from build123d import *

# Parameters (mm, degrees)
SKETCH1_R           = 31.75
SKETCH1_R_2         = 15.875
BOSS_EXTRUDE1_DEPTH = 82.55
BOSS_EXTRUDE2_DEPTH = 82.55
SKETCH4_R           = 9.525
CUT_EXTRUDE1_DEPTH  = 82.55
SKETCH5_W           = 19.05
SKETCH5_H           = 82.55
BOSS_EXTRUDE3_DEPTH = 88.9
CHAMFER1_SIZE       = 25.4
CUT_EXTRUDE2_REACH  = 211.476
SKETCH6_R           = 15.875


with BuildPart() as part:
    # Sketch1 → Boss-Extrude1 (new body)
    with BuildSketch(Plane.XY):
        Circle(SKETCH1_R)
        Circle(SKETCH1_R_2, mode=Mode.SUBTRACT)
    extrude(amount=-BOSS_EXTRUDE1_DEPTH)

    # Sketch3 → Boss-Extrude2 (add)
    with BuildSketch(Plane.XY):
        Polygon((0.997093544, 31.734339515), (-81.552906456, 31.734339515), (-81.552906456, 12.684339515), (-29.106185443, 12.684339515), align=None)
        Polygon((0, -31.75), (95.25, -31.75), (95.25, -12.7), (29.099355663, -12.7), align=None)
    extrude(amount=-BOSS_EXTRUDE2_DEPTH)

    # Sketch4 → Cut-Extrude1 (cut)
    with BuildSketch(Plane(origin=(0, 31.734339515, 0), x_dir=(1, 0, 0), z_dir=(0, 1, 0))):
        with Locations(Location((-56.152906456, 63.5, 0), (0, 0, 180))):
            Circle(SKETCH4_R)
        with Locations(Location((-56.152906456, 19.05, 0), (0, 0, 180))):
            Circle(SKETCH4_R)
    extrude(amount=-CUT_EXTRUDE1_DEPTH, mode=Mode.SUBTRACT)

    # Sketch5 → Boss-Extrude3 (add)
    with BuildSketch(Plane(origin=(0, -12.7, 0), x_dir=(1, 0, 0), z_dir=(0, 1, 0))):
        with Locations((85.725, 41.275)):
            Rectangle(SKETCH5_W, SKETCH5_H)
    extrude(amount=BOSS_EXTRUDE3_DEPTH)

    # Chamfer1
    chamfer1_edges = [part.edges().sort_by_distance(p)[0] for p in [
        (85.725, 76.2, -82.55),
        (85.725, 76.2, 0),
    ]]
    chamfer(chamfer1_edges, length=CHAMFER1_SIZE)

    # Sketch6 → Cut-Extrude2 (cut, up to next)
    with BuildSketch(Plane(origin=(95.25, 0, 0), x_dir=(0, 0, -1), z_dir=(1, 0, 0)), mode=Mode.PRIVATE) as cut_extrude2_sk1:
        with Locations((41.275, 19.05)):
            Circle(SKETCH6_R)
    cut_extrude2_tool1 = extrude(cut_extrude2_sk1.sketch, amount=-CUT_EXTRUDE2_REACH, mode=Mode.PRIVATE) & part.part
    add(cut_extrude2_tool1.solids().sort_by_distance((95.25, 19.05, -41.275))[0], mode=Mode.SUBTRACT)


solid = part.part
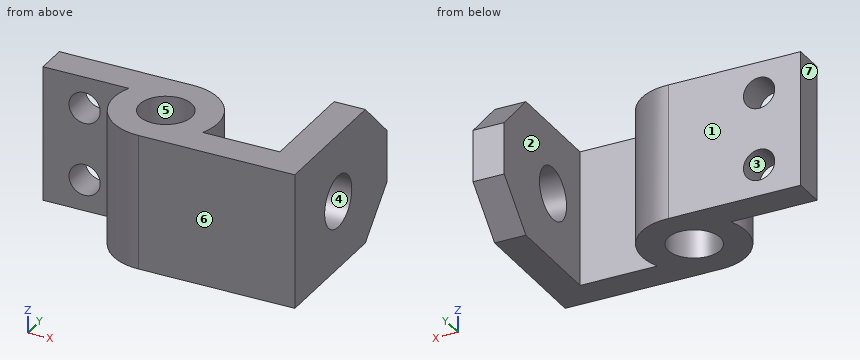
CAD build for the part. Positions are in the model's coordinates, mm. Face numbers are marked on the shaded views. A direction names the side the tool comes from. Round coordinates to 2 decimals unless told otherwise and drop trailing zeros. Write each loop counter-clockwise with the first axis right and the second up, starting at its lowest first coordinate (ties: lowest second). Pieces come first, ordered by that corner, then holes.
(1) 3-axis set-ups, long thin cutter, end or side, ignore diameter. For the marked faces 1, 2, 3 and 4: which of +Z, -Z, +X, -X, +Y, -Y reach the whole face in a straight line?
(2) Slice it at B-B, the plane z = -19.05. Write the cut outline in (x, y) (3 decimals).
(3) Slice it at A-A, the plane y = 19.05. Write the cut outline in (x, z) (3 decimals), and give its area (3 significant figures).
(4) Slice it at D-D, the plane z = -76.5. Write the cut outline in (x, y) (3 decimals).
(5) Slice it at C-C, the plane x = 11.5. Write the cut outline in (y, z), and give its area (3 significant figures).
(6) Probe line 1 along Y through (x, z) = (0, -54) (3 decimals); line 2 along X through (y, z) = (19.5, -16); line 3 along X through (y, z) = (3.5, -22). List the from-to ranges inside material, lowest first.
(7) Drop flat-ended pins along their axis: P1, Ø6, axis at x = -4.5, z = -52.5, coming from the +Y side; P2, Ø2, axis at x = -15.5, z = -39.5, coming from the -Y side; P3, Ø1, axis at x = -2, z = -39.5, coming from the -Y side. Give the stop position or say it passes through.
(8) Mould opens along X. For the marked faces 5, 6 and 7 say: pulls with the +X half, pulls with the -X half, needs draft (parallel to the pull), parting line crosses it, or undercut.
From the geometry:
1. face 1: +Z, -Z, -X, +Y
1. face 2: +Z, -Z, +Y
1. face 3: +Y, -Y
1. face 4: +X
2. outline: (-81.553, 12.684) - (-65.678, 12.684) - (-65.678, 31.734) - (-81.553, 31.734) - close; (-46.628, 12.684) - (-29.106, 12.684) arc R31.75 ccw to (0, -31.75) - (95.25, -31.75) - (95.25, 69.85) - (76.2, 69.85) - (76.2, -12.7) - (29.099, -12.7) arc R31.75 ccw to (-0.997, 31.734) - (-46.628, 31.734) - close; hole circle Ø31.75 at (0, 0)
3. outline: (-81.553, -82.55) - (25.4, -82.55) - (25.4, 0) - (-81.553, 0) - close; (76.2, -82.55) - (95.25, -82.55) - (95.25, -57.15) - (76.2, -57.15) - close; (76.2, -25.4) - (95.25, -25.4) - (95.25, 0) - (76.2, 0) - close; hole circle Ø19.05 at (-56.153, -63.5); hole circle Ø19.05 at (-56.153, -19.05)
3. area: 9,230 mm2
4. outline: (-81.553, 12.684) - (-29.106, 12.684) arc R31.75 ccw to (0, -31.75) - (95.25, -31.75) - (95.25, 56.85) - (76.2, 56.85) - (76.2, -12.7) - (29.099, -12.7) arc R31.75 ccw to (-0.997, 31.734) - (-81.553, 31.734) - close; hole circle Ø31.75 at (0, 0)
5. outline: (-31.75, -82.55) - (-10.94, -82.55) - (-10.94, 0) - (-31.75, 0) - close; (10.94, -82.55) - (29.59, -82.55) - (29.59, 0) - (10.94, 0) - close
5. area: 3,260 mm2
6. line 1: y = -31.75 to -15.875, 15.875 to 31.75
6. line 2: x = -81.55 to -65.18, -47.13 to 25.06, 76.2 to 95.25
6. line 3: x = -31.56 to -15.48, 15.48 to 31.56, 76.2 to 95.25
7. P1: stops at y = 31.73
7. P2: stops at y = -28.25
7. P3: stops at y = -31.71
8. face 5: undercut
8. face 6: needs draft
8. face 7: pulls with the -X half
